CAD build for the part. Positions are in the model's coordinates, mm. A direction names the side the tool comes from. Give positions to 0.01 mm unless a question says otherwise; leave off trailing zeros. Write each loop counter-clockwise with the first axis right and the second up, starting at its lowest first coordinate (ties: lowest second). Pieces come first, ordered by that corner, then holes. Notation, with made-up numbers: (47.25, -17.5) - (68.25, -17.5) arc R22 cw to (68.25, 1.5) - close; hole circle Ø4 at (-18, -26.5). An arc over 180 degrees is marked (long way). Answer as a JSON object with one key per item and string values.
from build123d import *

# Parameters (mm, degrees)
SKETCH1_R               = 5.35
BOSS_EXTRUDE2_DEPTH     = 7
BOSS_EXTRUDE3_START     = 8
SKETCH3_R               = 5.35
BOSS_EXTRUDE3_DEPTH     = 8
BOSS_EXTRUDE4_DEPTH     = 3
FILLET1_R               = 1
CHAMFER1_SIZE           = 10
CHAMFER2_SIZE           = 5
CUT_EXTRUDE1_DEPTH      = 67.560662475
CUT_EXTRUDE1_DEPTH_BACK = 67.560662475
SKETCH5_W               = 36.474956737
SKETCH5_H               = 3.5
SKETCH5_H_2             = 8
CHAMFER3_SIZE           = 7
SKETCH6_W               = 3
SKETCH6_H               = 7.094956055
SKETCH6_H_2             = 11.655043945
CUT_EXTRUDE2_DEPTH      = 3


# Some blends are built 0.0001 mm under size
with BuildPart() as part:
    # Sketch1 → Boss-Extrude2 (new body)
    with BuildSketch(Plane.XY):
        Polygon((-19.503784034, -20), (19.503784034, -20), (19.503784034, -18.25), (62.978740771, -18.25), (62.978740771, 13), (19.503784034, 13), (19.503784034, 20), (-19.503784034, 20), align=None)
        Circle(SKETCH1_R, mode=Mode.SUBTRACT)
    extrude(amount=-BOSS_EXTRUDE2_DEPTH)

    # Sketch3 → Boss-Extrude3 (add)
    with BuildSketch(Plane.XY.offset(BOSS_EXTRUDE3_START)):
        with BuildLine():
            Line((7.668115805, 5.35), (62.978740771, 5.35))
            Line((62.978740771, 5.35), (62.978740771, 9.35))
            Line((62.978740771, 9.35), (0, 9.35))
            ThreePointArc((0, 9.35), (-9.35, 0), (0, -9.35))
            Line((0, -9.35), (62.978740771, -9.35))
            Line((62.978740771, -9.35), (62.978740771, -5.35))
            Line((62.978740771, -5.35), (7.668115805, -5.35))
            ThreePointArc((7.668115805, -5.35), (9.35, 0), (7.668115805, 5.35))
        make_face()
        Circle(SKETCH3_R, mode=Mode.SUBTRACT)
    extrude(amount=-BOSS_EXTRUDE3_DEPTH)

    # Sketch4 → Boss-Extrude4 (add)
    with BuildSketch(Plane.XY):
        with BuildLine():
            Line((0, -18.25), (62.978740771, -18.25))
            Line((62.978740771, -18.25), (62.978740771, -16.25))
            Line((62.978740771, -16.25), (8.306623863, -16.25))
            Line((8.306623863, -16.25), (0, -16.25))
            ThreePointArc((0, -16.25), (-16.25, 0), (0, 16.25))
            Line((0, 16.25), (0, 18.25))
            ThreePointArc((0, 18.25), (-18.25, 0), (0, -18.25))
        make_face()
    extrude(amount=BOSS_EXTRUDE4_DEPTH)

    # Fillet1
    fillet1_edges = [part.edges().sort_by_distance(p)[0] for p in [
        (0, 16.25, 1.5),
        (0, 18.25, 1.5),
    ]]
    fillet(fillet1_edges, radius=FILLET1_R - 0.0001)  # a hair under: the kernel refuses the full size

    # Chamfer1
    # the kernel refuses this chamfer: 10 mm, written as the material it takes off along each edge
    with BuildSketch(Plane(origin=(19.503784034, -20, 25.71682988), x_dir=(0.027495876610586317, 0.9996219169112968, 0), z_dir=(0, 0, -1))) as chamfer1_piece_1_section:
        Polygon((CHAMFER1_SIZE * 0.999621916911, -CHAMFER1_SIZE * 0.0274958766106), (-CHAMFER1_SIZE * 0.0274958766106, -CHAMFER1_SIZE * 0.999621916911), (0, 0), align=None)
    chamfer1_piece_1 = extrude(amount=58.433659759, mode=Mode.PRIVATE)
    chamfer1_piece_1 = split(chamfer1_piece_1, bisect_by=Plane(origin=(14.814200223, -18.25, -3.5), z_dir=(0, -1, 0)), keep=Keep.TOP, mode=Mode.PRIVATE)
    add(chamfer1_piece_1, mode=Mode.SUBTRACT)

    # Chamfer2
    chamfer2_edges = [part.edges().sort_by_distance(p)[0] for p in [
        (-19.503784034, -20, -3.5),
        (-19.503784034, 20, -3.5),
    ]]
    chamfer(chamfer2_edges, length=CHAMFER2_SIZE)

    # Sketch5 → Cut-Extrude1 (cut, two sides: drawn at the far end of the back side and taken through both)
    with BuildSketch(Plane.XY.offset(-CUT_EXTRUDE1_DEPTH_BACK)):
        with Locations((37.741262403, 3.6)):
            Rectangle(SKETCH5_W, SKETCH5_H)
        with Locations((37.741262403, -7.15)):
            Rectangle(SKETCH5_W, SKETCH5_H_2)
    extrude(amount=CUT_EXTRUDE1_DEPTH + CUT_EXTRUDE1_DEPTH_BACK, mode=Mode.SUBTRACT)

    # Chamfer3
    chamfer3_edges = [part.edges().sort_by_distance(p)[0] for p in [
        (19.503784034, 20, -3.5),
    ]]
    chamfer(chamfer3_edges, length=CHAMFER3_SIZE - 0.0001)  # a hair under: the kernel refuses the full size

    # Sketch6 → Cut-Extrude2 (cut)
    with BuildSketch(Plane(origin=(62.978740771, 0, 0), x_dir=(0, 0, -1), z_dir=(1, 0, 0))):
        with Locations((3.5, 6.452521972)):
            Rectangle(SKETCH6_W, SKETCH6_H)
        with Locations((3.5, -8.922478028)):
            Rectangle(SKETCH6_W, SKETCH6_H_2)
    extrude(amount=-CUT_EXTRUDE2_DEPTH, mode=Mode.SUBTRACT)


solid = part.part
(1) 3-axis set-ups, long thin cutter, end or side, ignore diameter. For faces 1 (the face through (35, 5.35, 1)), 2 (the face through (19.504, 4, -4)), 3 (the face through (-1, 20, -3)), 4 (the face through (61, -3.095, -3)), 5 (the face through (60, -5.35, 4)): which of +Z, -Z, +X, -X, +Y, -Y reach the whole face in a straight line?
Answer key:
{"face 1": "+Z", "face 2": "+Z, -Z", "face 3": "+Z, -Z, +X, -X, +Y", "face 4": "+X", "face 5": "+Z, +X"}
(2) Probe L1, parallel to Y at x = 16, z = 2; L2, parallel to Y at x = 21.5, z = -3; L3, parallel to Y at x = 16.5, z = 3.25. List the from-to ranges inside material, lowest first. Write a range as [from, to].
Answer key:
{"L1": "y = [-18.25, -16.25], [-9.35, -5.35], [5.35, 9.35]", "L2": "y = [-18.25, -11.15], [-3.15, 1.85], [5.35, 13]", "L3": "y = [-9.35, -5.35], [5.35, 9.35]"}
(3) Pull direction Y, two halves, no side cores. Call faces 6 (the face through (-17.039, 17.465, -3.451)), 7 (the face through (12, 0, -7)), 8 (the face through (55.979, -7, -1)): pulls with the +Y half, pulls with the -Y half, needs draft (parallel to the pull), parting line crosses it, or undercut.
Answer key:
{"face 6": "pulls with the +Y half", "face 7": "needs draft", "face 8": "undercut"}
(4) Saw through at A-A, the plane z = 1.5. State how many separate pieces and enclosed holes the cut face has, and give its area (3 significant figures).
Answer key:
{"separate pieces": "3", "enclosed holes": "1", "area": "734 mm²"}
(5) Flat gauge pins, fed straight in: P1, Ø0.9, axis at y = 5.5, z = -4, coming from the +X side; P2, Ø3.5, axis at x = 44, z = -3, coming from the +Y side; P3, Ø0.9, axis at x = 61.5, y = -10, coming from the +Z side. Where does each tip first touch, or does it go through?
Answer key:
{"P1": "stops at x = 59.98", "P2": "stops at y = 13", "P3": "stops at z = 0"}
(6) Saw through at C-C, the plane z = 5.5. Give the cut face in (x, y).
Answer key:
{"outline": "(0, -9.35) - (19.5, -9.35) - (19.5, -5.35) - (7.67, -5.35) arc R9.35 ccw to (7.67, 5.35) - (62.98, 5.35) - (62.98, 9.35) - (0, 9.35) arc R9.35 ccw to start; (55.98, -9.35) - (62.98, -9.35) - (62.98, -5.35) - (55.98, -5.35) - close; hole circle Ø10.7 at (0, 0)"}
(7) Saw through at B-B, the plane y = 0. Give the cut face in (x, z).
Answer key:
{"outline": "(-19.5, -7) - (-5.35, -7) - (-5.35, 8) - (-9.35, 8) - (-9.35, 0) - (-16.25, 0) - (-16.25, 3) - (-18.25, 3) - (-18.25, 0) - (-19.5, 0) - close; (5.35, -7) - (62.98, -7) - (62.98, 0) - (9.35, 0) - (9.35, 8) - (5.35, 8) - close"}
(8) Saw through at D-D, the plane x = 54. Give the cut face in (y, z), and give its area (3 significant figures).
Answer key:
{"outline": "(-18.25, -7) - (-11.15, -7) - (-11.15, 0) - (-16.25, 0) - (-16.25, 3) - (-18.25, 3) - close; (-3.15, -7) - (1.85, -7) - (1.85, 0) - (-3.15, 0) - close; (5.35, -7) - (13, -7) - (13, 0) - (9.35, 0) - (9.35, 8) - (5.35, 8) - close", "area": "176 mm²"}
